Model file for the job. Use its own axes, mm. Round coordinates to 2 decimals unless told otherwise and drop trailing zeros. Write each loop counter-clockwise with the first axis right and the second up, starting at its lowest first coordinate (ties: lowest second). Pieces come first, ordered by that corner, then holes. Notation, with made-up numbers: (-8.5, -29.75) - (14.5, -29.75) arc R7 cw to (14.5, -23.75) - close; hole circle Ø9 at (64, 6). An arc over 180 degrees is marked (long way). One line per item, written item: value.
from build123d import *

# Parameters (mm, degrees)
SKETCH1_W             = 76
SKETCH1_H             = 38.238165328
SKETCH1_R             = 1.27
BOSS_EXTRUDE1_DEPTH   = 6.35
F_8_0MM_DOWEL_HOLE1_D = 8


with BuildPart() as part:
    # Sketch1 → Boss-Extrude1 (new body)
    with BuildSketch(Plane.XY):
        with Locations((38, 23.427645759)):
            Rectangle(SKETCH1_W, SKETCH1_H)
        with Locations((18, 24.308563095)):
            Circle(SKETCH1_R, mode=Mode.SUBTRACT)
        with Locations((58, 24.308563095)):
            Circle(SKETCH1_R, mode=Mode.SUBTRACT)
    extrude(amount=BOSS_EXTRUDE1_DEPTH)

    # Ø8.0mm Dowel Hole1 (through all)
    with Locations(Plane.XY.offset(6.35)):
        with Locations((18, 24.308563095), (58, 24.308563095)):
            Hole(F_8_0MM_DOWEL_HOLE1_D / 2)


solid = part.part
1. Band-saw the part on B-B on z = 5.5. Write the cut outline in (x, y).
Report:
outline: (0, 4.31) - (76, 4.31) - (76, 42.55) - (0, 42.55) - close; hole circle Ø8 at (18, 24.31); hole circle Ø8 at (58, 24.31)
2. Mould opens along X. For faces 1 (the face through (18.867, 20.404, 3.131)), 2 (the face through (54.305, 22.777, 3.131)), 3 (the face through (76, 23, 3)), 4 (the face through (37, 4.309, 3)) say: released by +X, released by -X, zero draft, split by the parting line, or undercut.
Report:
face 1: undercut
face 2: undercut
face 3: released by +X
face 4: zero draft
3. Wall check: probe 1 along X at (y, z) = (27, 2.5); probe 2 along X at (y, z) = (24, 5); probe 3 along Y at (x, z) = (58, 1.75). Give the ranges that are in metal, low to high. Write a range as [from, to].
Report:
probe 1: [0, 15.04], [20.96, 55.04], [60.96, 76]
probe 2: [0, 14.01], [21.99, 54.01], [61.99, 76]
probe 3: [4.31, 20.31], [28.31, 42.55]
4. Band-saw the part on A-A on x = 18. Write the cut outline in (y, z), plus the area to 3 significant figures.
Report:
outline: (4.31, 0) - (20.31, 0) - (20.31, 6.35) - (4.31, 6.35) - close; (28.31, 0) - (42.55, 0) - (42.55, 6.35) - (28.31, 6.35) - close
area: 192 mm²
